Can you work these out from the drawing? Everything is in mm from the part's minimum corner. A direction names the side the tool comes from. Round coordinates to 2 decimals unless told otherwise and drop trailing zeros. Order: outer loops, then holes, each group sorted by start corner. A loop starts at its lowest first (then second) coordinate and runs counter-clockwise, first axis right, second up. Notation, with made-up numbers: M 89.25,15 L 135.25,15 A6 ccw 135.25,25 Z; hole C 61,88 d10. An arc over 180 degrees is marked long. Answer as a JSON object with one key per item and string values. Group by question number.
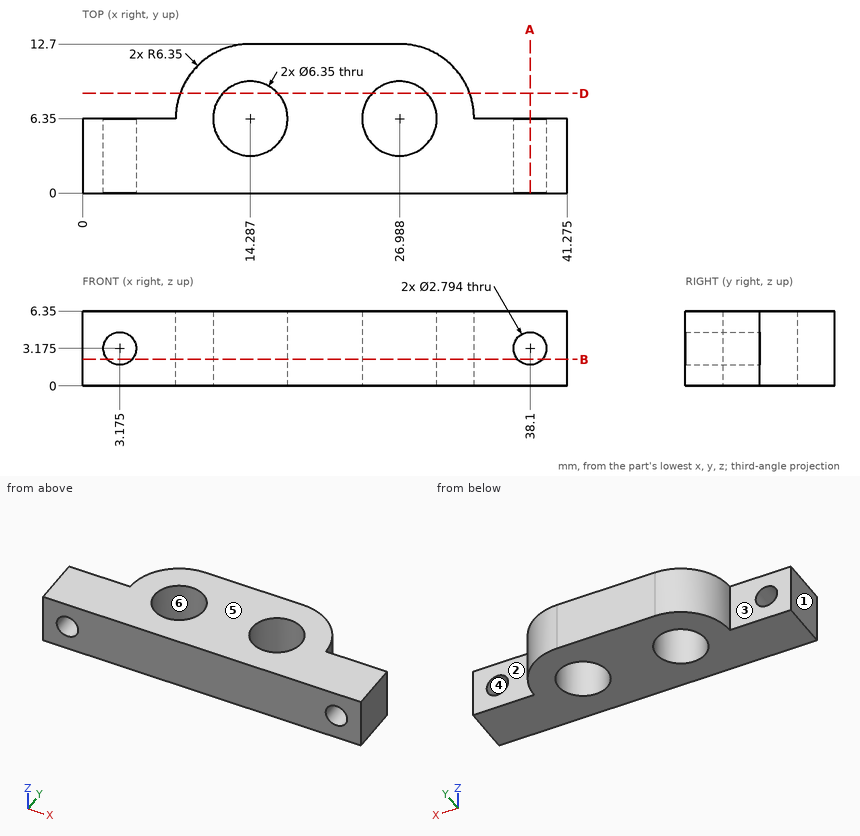
Item 1: I'm going to push flat-ended pins straight in: pin 1 Ø2 at (y, z) = (10.5, 1) entering from +X; pin 2 Ø1 at (x, z) = (6, 3.5) entering from +Y; pin 3 Ø2 at (y, z) = (7.5, 5.5) entering from +X; pin 4 Ø5 at (x, y) = (14.29, 6.35) entering from -Z. Where does each tip first touch, or does it pass through?
Item 2: Suppose I cut it at A-A, the plane x = 38.1. Write out the boundary of the cut face in (y, z).
Item 3: I need wall thicknesses on line 1 (X direction, y = 4.5, z = 4.75) (1 decimal); line 2 (X direction, y = 7.25, z = 2.5); line 3 (Z direction, x = 38.1, y = 5.25). Which ranges of each line are inside material? Lowest first, please.
Item 4: If we mould it in two halves opening along Z, with no side actions, what happens to the marked faces 4, 5 and 6? For each: +Z half, -Z half, draft (parallel to the pull), parting line (faces both ways), or undercut.
Item 5: Suppose I cut it at D-D, the plane y = 8.5. Write out the boundary of the cut face in (x, z).
Item 6: On a 3-axis mill with a long thin cutter (end or side, diameter ignored), from which of +Z, -Z, +X, -X, +Y, -Y can I reach the whole of each face in a straight line? I mean the marked faces 1, 2 and 3. Say none if no direction works.
Item 7: Suppose I cut it at B-B, the plane z = 2.25. State how many separate pieces and enclosed holes the cut face has, and give its area (3 significant figures).
Computed:
{
 "1": {"pin 1": "stops at x = 32.5", "pin 2": "stops at y = 6.35", "pin 3": "stops at x = 33.34", "pin 4": "passes through"},
 "2": {"outline": "M 0,0 L 6.35,0 L 6.35,1.78 L 0,1.78 Z; M 0,4.57 L 6.35,4.57 L 6.35,6.35 L 0,6.35 Z"},
 "3": {"line 1": "x = 0 to 11.7, 16.9 to 24.4, 29.6 to 41.3", "line 2": "x = 8 to 11.24, 17.33 to 23.94, 30.03 to 33.27", "line 3": "z = 0 to 1.78, 4.57 to 6.35"},
 "4": {"face 4": "undercut", "face 5": "+Z half", "face 6": "draft"},
 "5": {"outline": "M 8.31,0 L 11.95,0 L 11.95,6.35 L 8.31,6.35 Z; M 16.62,0 L 24.65,0 L 24.65,6.35 L 16.62,6.35 Z; M 29.32,0 L 32.96,0 L 32.96,6.35 L 29.32,6.35 Z"},
 "6": {"face 1": "+Z, -Z, -X, +Y, -Y", "face 2": "+Z, -Z, +X, +Y", "face 3": "+Z, -Z, -X, +Y"},
 "7": {"separate pieces": "3", "enclosed holes": "2", "area": "316 mm^2"}
}
